Design review of the part built by this model. Coordinates are the model's own, in mm. Face numbers are marked on the shaded views. A direction names the side the tool comes from. Give positions to 0.01 mm unless a question says otherwise; leave off trailing zeros. Write each loop counter-clockwise with the first axis right and the second up, starting at its lowest first coordinate (ties: lowest second). Pieces come first, ordered by that corner, then holes.
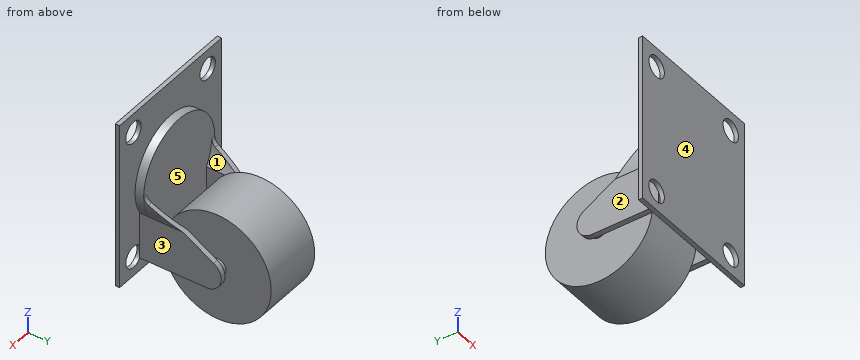
```python
from build123d import *
from build123d.topology import SkipClean

# Parameters (mm, degrees)
SKETCH1_W               = 33
SKETCH1_H               = 39
SKETCH1_R               = 2.5
BOSS_EXTRUDE1_DEPTH     = 1
BOSS_EXTRUDE2_DEPTH     = 2
BOSS_EXTRUDE3_START     = -17
BOSS_EXTRUDE3_DEPTH     = 17
CUT_EXTRUDE1_DEPTH      = 39.503246616
CUT_EXTRUDE1_DEPTH_BACK = 39.503246616


with BuildPart() as part:
    # Sketch1 → Boss-Extrude1 (new body)
    with BuildSketch(Plane(origin=(0, 0, 0), x_dir=(1, 0, 0), z_dir=(0, 1, 0))):
        Rectangle(SKETCH1_W, SKETCH1_H)
        with Locations(Location((12, -15, 0), (0, 0, 270))):
            Circle(SKETCH1_R, mode=Mode.SUBTRACT)
        with Locations(Location((-12, -15, 0), (0, 0, 270))):
            Circle(SKETCH1_R, mode=Mode.SUBTRACT)
        with Locations(Location((-12, 15, 0), (0, 0, 270))):
            Circle(SKETCH1_R, mode=Mode.SUBTRACT)
        with Locations(Location((12, 15, 0), (0, 0, 270))):
            Circle(SKETCH1_R, mode=Mode.SUBTRACT)
    extrude(amount=BOSS_EXTRUDE1_DEPTH)

    # Sketch2 → Boss-Extrude2 (add)
    with BuildSketch(Plane(origin=(0, 1, 0), x_dir=(1, 0, 0), z_dir=(0, 1, 0))):
        with BuildLine():
            Line((10, 5.678908346), (10, 16.5))
            Line((10, 16.5), (-10, 16.5))
            Line((-10, 16.5), (-10, 5.678908346))
            ThreePointArc((-10, 5.678908346), (0, -11.5), (10, 5.678908346))
        make_face()
    extrude(amount=BOSS_EXTRUDE2_DEPTH)

    # Sketch3 → Boss-Extrude3 (add)
    with SkipClean():  # the faces are left unmerged after this step: merging them gives an invalid solid
        with BuildSketch(Plane(origin=(0, 20, 0), x_dir=(1, 0, 0), z_dir=(0, 1, 0)).offset(BOSS_EXTRUDE3_START)):
            with BuildLine():
                Line((-10.466352676, 0), (-11.5, 0))
                ThreePointArc((-11.5, 0), (-11.118677979, 2.936835031), (-10, 5.678908346))
                Line((-10, 5.678908346), (-10, 16.5))
                Line((-10, 16.5), (-8.791731248, 16.5))
                Line((-8.791731248, 16.5), (-8.791731248, 5.678908346))
                ThreePointArc((-8.791731248, 5.678908346), (-10.038971516, 2.960336), (-10.466352676, 0))
            make_face()
            with BuildLine():
                Line((8.791731248, 16.5), (8.791731248, 5.678908346))
                ThreePointArc((8.791731248, 5.678908346), (10.038971516, 2.960336), (10.466352676, 0))
                Line((10.466352676, 0), (11.5, 0))
                ThreePointArc((11.5, 0), (11.118677979, 2.936835031), (10, 5.678908346))
                Line((10, 5.678908346), (10, 16.5))
                Line((10, 16.5), (8.791731248, 16.5))
            make_face()
        extrude(amount=BOSS_EXTRUDE3_DEPTH)

    # Sketch4 → Cut-Extrude1 (cut, two sides: drawn at the far end of the back side and taken through both)
    with SkipClean():  # the faces are left unmerged after this step: merging them gives an invalid solid
        with BuildSketch(Plane(origin=(10, 0, 0), x_dir=(0, 0, -1), z_dir=(1, 0, 0)).offset(-CUT_EXTRUDE1_DEPTH_BACK)):
            with BuildLine():
                Line((-2.613781241, 3), (-0.185143028, 3))
                ThreePointArc((-0.185143028, 3), (0.810549083, 3.265469165), (1.541915642, 3.991402781))
                Line((1.541915642, 3.991402781), (9.859295901, 18.23356349))
                ThreePointArc((9.859295901, 18.23356349), (13.867346815, 19.876273461), (16.5, 16.436490709))
                Line((16.5, 16.436490709), (17.783999393, 20))
                Line((17.783999393, 20), (0.550387099, 24.196515301))
                Line((0.550387099, 24.196515301), (-11.381791723, 8.604740189))
                Line((-11.381791723, 8.604740189), (-2.613781241, 3))
            make_face()
        extrude(amount=CUT_EXTRUDE1_DEPTH + CUT_EXTRUDE1_DEPTH_BACK, mode=Mode.SUBTRACT)

    # Sketch5 → Revolve1 (revolve)
    with SkipClean():  # the faces are left unmerged after this step: merging them gives an invalid solid
        with BuildSketch(Plane(origin=(0, 17, 0), x_dir=(1, 0, 0), z_dir=(0, 1, 0)), mode=Mode.PRIVATE) as revolve1_sk:
            Polygon((7.035069501, 11.179647951), (8.791731248, 11.179647951), (8.791731248, 13.179647951), (0, 13.179647951), (0, 0.679647951), (7.035069501, 0.679647951), align=None)
            Polygon((0, 0.679647951), (0, 13.179647951), (-8.791731248, 13.179647951), (-8.791731248, 11.179647951), (-7.035069501, 11.179647951), (-7.035069501, 0.679647951), align=None)
        revolve(revolve1_sk.sketch.rotate(Axis((8.791731248, 17, -13.179647951), (-1, 0, 0)), 180), axis=Axis((8.791731248, 17, -13.179647951), (-1, 0, 0)))


solid = part.part
```
(1) Consider section C-C, the plane x = -4. Give the boundary of the cut face in (y, z).
Resolved:
outline: (0, -19.5) - (1, -19.5) - (1, -16.5) - (3, -16.5) - (3, 10.78) - (1, 10.78) - (1, 19.5) - (0, 19.5) - close; circle Ø25 at (17, -13.18)
(2) Clearance check with flat-ended pins moving along their axes: P1, Ø3, axis at y = 14.5, z = -9, coming from the -X side; P2, Ø5, axis at x = 4, y = 20.5, coming from the +Z side; P3, Ø6, axis at x = -9, y = 7, coming from the -Z side; P4, Ø4.5, axis at x = 12, z = 15, coming from the +Y side. State where each tip first meets the part, or that it passes through.
Resolved:
P1: stops at x = -10
P2: stops at z = -0.72
P3: stops at z = -23
P4: passes through
(3) Consider section A-A, the plane x = 13.5. Give the boundary of the cut face in (y, z), then the cut area to 3 significant figures.
Resolved:
outline: (0, -19.5) - (1, -19.5) - (1, -17) - (0, -17) - close; (0, -13) - (1, -13) - (1, 13) - (0, 13) - close; (0, 17) - (1, 17) - (1, 19.5) - (0, 19.5) - close
area: 31.0 mm2
(4) To check wall thickness, follow L1, parallel to X at y = 7, z = -6.5; L2, parallel to X at y = 0.5, z = 15; L3, parallel to X at y = 4.75, z = -8. State the ranges of each line that lie inside material, in increasing order.
Resolved:
L1: x = -10 to -8.79, -7.04 to 7.04, 8.79 to 10
L2: x = -16.5 to -14.5, -9.5 to 9.5, 14.5 to 16.5
L3: x = -10 to -8.79, 8.79 to 10
(5) Consider section B-B, the plane z = 15. Give the boundary of the cut face in (x, y), then the cut area to 3 significant figures.
Resolved:
outline: (-16.5, 0) - (-14.5, 0) - (-14.5, 1) - (-16.5, 1) - close; (-9.5, 0) - (9.5, 0) - (9.5, 1) - (-9.5, 1) - close; (14.5, 0) - (16.5, 0) - (16.5, 1) - (14.5, 1) - close
area: 23.0 mm2
(6) Consider section D-D, the plane z = 8. Give the boundary of the cut face in (x, y).
Resolved:
outline: (-16.5, 0) - (16.5, 0) - (16.5, 1) - (8.26, 1) - (8.26, 3) - (-8.26, 3) - (-8.26, 1) - (-16.5, 1) - close
(7) Mouldability with a two-part tool opening along Y and no side actions: class the marked faces 3, 4 and 5 as pulls with the +Y half, pulls with the -Y half, needs draft (parallel to the pull), parting line crosses it, or undercut.
Resolved:
face 3: needs draft
face 4: pulls with the -Y half
face 5: undercut
(8) Tool access review of the marked faces 1 and 2: name each direction out of +Z, -Z, +X, -X, +Y, -Y from which nothing blocks a thin tool from reaching the whole face with its end or side.
Resolved:
face 1: +Z, +Y
face 2: -Z, -X, +Y
